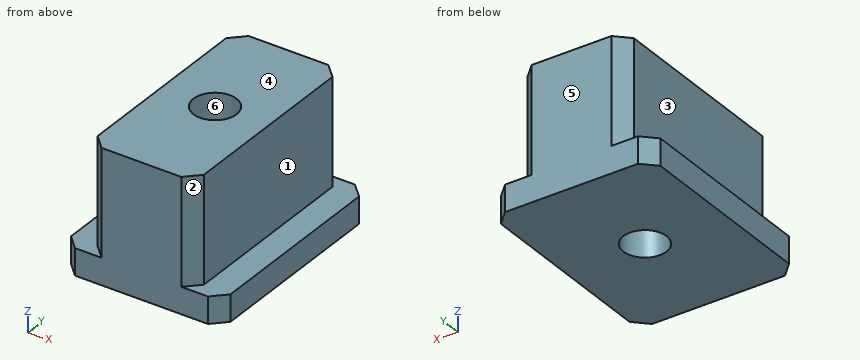
Autodesk Inventor part; units mm, degrees
ref_plane "YZ Plane" through (0, 0, 0) normal (1, 0, 0) x (0, 1, 0)
ref_plane "XZ Plane" through (0, 0, 0) normal (0, 1, 0) x (-1, 0, 0)
ref_plane "XY Plane" through (0, 0, 0) normal (0, 0, 1) x (1, 0, 0)
sketch "Esboço1" plane through (0, 0, 0) normal (0, 0, 1) x (1, 0, 0)
  line L0 (-6, 8) -> (6, 8)
  line L1 (6, 8) -> (6, -8)
  line L2 (6, -8) -> (-6, -8)
  line L3 (-6, -8) -> (-6, 8)
  line L4 (-6, 8) -> (6, -8) construction
  line L5 (6, 8) -> (-6, -8) construction
  point P0 (0, 0)
  dimension "d0" = 12
  dimension "d1" = 16
extrude "Extrusão1" add sketch "Esboço1" along normal blind 10
sketch "Esboço3" plane through (0, 0, 10) normal (0, 0, 1) x (1, 0, 0)
  line L0 (6, -8) -> (-6, -8)
  line L1 (-6, -8) -> (-6, 8)
  line L2 (-6, 8) -> (6, 8)
  line L3 (6, 8) -> (6, -8)
  line L4 (6, -8) -> (-6, 8) construction
  line L5 (-6, -8) -> (6, 8) construction
  line L6 (4, -8) -> (-4, -8)
  line L7 (-4, -8) -> (-4, 8)
  line L8 (-4, 8) -> (4, 8)
  line L9 (4, 8) -> (4, -8)
  line L10 (4, -8) -> (-4, 8) construction
  line L11 (-4, -8) -> (4, 8) construction
  point P0 (0, 0)
  dimension "d4" = 12
  dimension "d5" = 16
  dimension "d6" = 8
extrude "Extrusão2" cut sketch "Esboço3" against normal blind 8 contours L0 L9 L2 L3 | L0 L1 L2 L7
chamfer "Chanfro1" distance 1 angle 45 8 edges at (6, -8, 1) (-6, -8, 1) (6, 8, 1) (-6, 8, 1) (-4, -8, 6) (-4, 8, 6) (4, 8, 6) (4, -8, 6)
sketch "Esboço4" plane through (0, 0, 10) normal (0, 0, 1) x (1, 0, 0)
  circle A0 centre (0, 0) radius 1.5 construction
  dimension "d12" = 3
hole "Furo1" at (0, 0, 10) direction (0, 0, -1) diameter 3.242 end through all
Input: part model. Units: mm. Frame: model coordinates. Face numbers are marked on the shaded views. A direction names the side the tool comes from. Give positions to 0.01 mm unless a question says otherwise; leave off trailing zeros. Write each loop counter-clockwise with the first axis right and the second up, starting at its lowest first coordinate (ties: lowest second). Pieces come first, ordered by that corner, then holes. Notation, with made-up numbers: (35.5, -25) - (89.5, -25) arc R16 cw to (89.5, -6) - close; hole circle Ø7 at (41.5, 66). An arc over 180 degrees is marked (long way). Write item = value, one per line. Start each with the question number.
1. First-contact query: pin 1 Ø2.5 at (y, z) = (-1, 4.5) entering from +X; pin 2 Ø2 at (y, z) = (-5, 3.5) entering from -X. Flat tips, straight axial feed; report the tip coordinate or a pass-through.
2. Section query D-D, the plane y = -6.5. Output: boundary loops of the cut face in (x, z), then the cut area to 3 significant figures.
3. Section query B-B, the plane y = 0. Output: boundary loops of the cut face in (x, z), then the cut area to 3 significant figures.
4. Section query C-C, the plane z = 9.25. Output: boundary loops of the cut face in (x, y), then the cut area to 3 significant figures.
5. Section query A-A, the plane x = 0. Output: boundary loops of the cut face in (y, z), then the cut area to 3 significant figures.
6. Access query for the marked faces 1, 2 and 3. Directions: +Z, -Z, +X, -X, +Y, -Y. A direction counts if a zero-diameter tool reaches every point of the face in a straight line with its end or side. Return the directions, or none.
7. Ray query, L1, parallel to X at y = 0, z = 5.5; L2, parallel to Y at x = 0, z = 7; L3, parallel to X at y = -6, z = 3. Return the intervals inside material, ascending.
8. Mould query, pull axis Y, two halves, no side actions, for the marked faces 4, 5 and 6. Classes: released by +Y, released by -Y, zero draft, split by the parting line, or undercut.
Check sheet entries:
q1.pin_1 = 4
q1.pin_2 = -4
q2.outline = (-6, 0) - (6, 0) - (6, 2) - (4, 2) - (4, 10) - (-4, 10) - (-4, 2) - (-6, 2) - close
q2.area = 88.0 mm2
q3.outline = (-6, 0) - (-1.62, 0) - (-1.62, 10) - (-4, 10) - (-4, 2) - (-6, 2) - close; (1.62, 0) - (6, 0) - (6, 2) - (4, 2) - (4, 10) - (1.62, 10) - close
q3.area = 55.6 mm2
q4.outline = (-4, -7) - (-3, -8) - (3, -8) - (4, -7) - (4, 7) - (3, 8) - (-3, 8) - (-4, 7) - close; hole circle Ø3.24 at (0, 0)
q4.area = 118 mm2
q5.outline = (-8, 0) - (-1.62, 0) - (-1.62, 10) - (-8, 10) - close; (1.62, 0) - (8, 0) - (8, 10) - (1.62, 10) - close
q5.area = 128 mm2
q6.face_1 = +Z, +X, +Y, -Y
q6.face_2 = +Z, +X, -Y
q6.face_3 = +Z, -X, +Y, -Y
q7.L1 = -4 to -1.62, 1.62 to 4
q7.L2 = -8 to -1.62, 1.62 to 8
q7.L3 = -4 to 4
q8.face_4 = zero draft
q8.face_5 = released by +Y
q8.face_6 = undercut
